Geometry: final body of the model. Coordinates: model frame, mm. A direction names the side the tool comes from. Give positions to 0.01 mm unless a question says otherwise; leave off trailing zeros. Loops run counter-clockwise (first coordinate to the right, second up) from the corner with the lowest first, then second, coordinate; pieces in that order, holes last.
1. Section B-B, the plane y = 1.15. Output: boundary loops of the cut face in (x, z).
2. Draft query along X for faces 1 (the face through (-67.25, 2, -46)), 2 (the face through (65.436, 1.61, -90.045)), 3 (the face through (-20.63, 1.57, -39.96)), 4 (the face through (20.63, 1.57, -85.24)). Return one class per face: +X half, -X half, draft (parallel to the pull), parting line (faces both ways), or undercut.
3. Section D-D, the plane x = 27.5. Output: boundary loops of the cut face in (y, z) (1 decimal), then the cut area to 3 significant figures.
4. Section A-A, the plane z = -42.6. Output: boundary loops of the cut face in (x, y) (3 decimals), then the cut area to 3 significant figures.
5. Material intervals for line 1 along X through (y, z) = (1.15, -43); line 2 along X through (y, z) = (0.65, -41); line 3 along X through (y, z) = (0.1, -69), sorted ascending.
6. Section C-C, the plane x = 44.5. Output: boundary loops of the cut face in (y, z) (3 decimals).
7. Access query for faces 5 (the face through (-1, 3.175, -29)), 6 (the face through (29.8, 1.6, -62.9)). Directions: +Z, -Z, +X, -X, +Y, -Y. A direction counts if a zero-diameter tool reaches every point of the face in a straight line with its end or side. Return the directions, or none.
8. First-contact query: P1, Ø4, axis at x = -51, z = -69.1, coming from the -Y side; P2, Ø1, axis at x = 2, y = 1, coming from the -Z side. Flat tips, straight axial feed; report the tip coordinate or a pass-through.
from build123d import *

# Parameters (mm, degrees)
SKETCH1_R           = 2.5
SKETCH1_R_2         = 12.25
BOSS_EXTRUDE1_DEPTH = 3.175
FILLET1_R           = 9.2
FILLET2_R           = 6.7


with BuildPart() as part:
    # Sketch1 → Boss-Extrude1 (new body)
    with BuildSketch(Plane(origin=(0, 0, 0), x_dir=(1, 0, 0), z_dir=(0, 1, 0))):
        with BuildLine():
            Line((-67.25, 0), (67.25, 0))
            Line((67.25, 0), (67.25, 91.408280206))
            ThreePointArc((67.25, 91.408280206), (0, 101.8), (-67.25, 91.408280206))
            Line((-67.25, 91.408280206), (-67.25, 0))
        make_face()
        with Locations(Location((-51, 69.1, 0), (0, 0, 270))):
            Circle(SKETCH1_R, mode=Mode.SUBTRACT)
        with Locations(Location((51, 69.1, 0), (0, 0, 270))):
            Circle(SKETCH1_R, mode=Mode.SUBTRACT)
        with Locations(Location((0, 12.1, 0), (0, 0, 270))):
            Circle(SKETCH1_R, mode=Mode.SUBTRACT)
        with Locations(Location((42, 42.6, 0), (0, 0, 270))):
            Circle(SKETCH1_R_2, mode=Mode.SUBTRACT)
        with BuildLine():
            Line((-14.622204703, 86.85), (14.622204703, 86.85))
            ThreePointArc((14.622204703, 86.85), (20.704967234, 85.194080433), (25.108968848, 80.683333333))
            ThreePointArc((25.108968848, 80.683333333), (29.8, 62.6), (25.108968848, 44.516666667))
            ThreePointArc((25.108968848, 44.516666667), (20.704967234, 40.005919567), (14.622204703, 38.35))
            Line((14.622204703, 38.35), (-14.622204703, 38.35))
            ThreePointArc((-14.622204703, 38.35), (-20.704967234, 40.005919567), (-25.108968848, 44.516666667))
            ThreePointArc((-25.108968848, 44.516666667), (-29.8, 62.6), (-25.108968848, 80.683333333))
            ThreePointArc((-25.108968848, 80.683333333), (-20.704967234, 85.194080433), (-14.622204703, 86.85))
        make_face(mode=Mode.SUBTRACT)
    extrude(amount=BOSS_EXTRUDE1_DEPTH)

    # Fillet1
    fillet1_edges = [part.edges().sort_by_distance(p)[0] for p in [
        (-67.25, 1.5875, -91.408280206),
        (67.25, 1.5875, -91.408280206),
    ]]
    fillet(fillet1_edges, radius=FILLET1_R)

    # Fillet2
    fillet2_edges = [part.edges().sort_by_distance(p)[0] for p in [
        (67.25, 1.5875, 0),
        (-67.25, 1.5875, 0),
    ]]
    fillet(fillet2_edges, radius=FILLET2_R)


solid = part.part
Answers below:
1. outline: (-67.25, -84.56) arc R9.2 ccw to (-60.55, -93.41) arc R222.8 ccw to (60.55, -93.41) arc R9.2 ccw to (67.25, -84.56) - (67.25, -6.7) arc R6.7 ccw to (60.55, 0) - (-60.55, 0) arc R6.7 ccw to (-67.25, -6.7) - close; hole circle Ø5 at (-51, -69.1); hole (-25.11, -80.68) arc R12 ccw to (-14.62, -86.85) - (14.62, -86.85) arc R12 ccw to (25.11, -80.68) arc R37.2 ccw to (25.11, -44.52) arc R12 ccw to (14.62, -38.35) - (-14.62, -38.35) arc R12 ccw to (-25.11, -44.52) arc R37.2 ccw to start; hole circle Ø5 at (0, -12.1); hole circle Ø24.5 at (42, -42.6); hole circle Ø5 at (51, -69.1)
2. face 1: -X half
2. face 2: +X half
2. face 3: undercut
2. face 4: undercut
3. outline: (0, -100.1) - (3.2, -100.1) - (3.2, -75.5) - (0, -75.5) - close; (0, -49.7) - (3.2, -49.7) - (3.2, 0) - (0, 0) - close
3. area: 236 mm2
4. outline: (-67.25, 0) - (-23.784, 0) - (-23.784, 3.175) - (-67.25, 3.175) - close; (23.784, 0) - (29.75, 0) - (29.75, 3.175) - (23.784, 3.175) - close; (54.25, 0) - (67.25, 0) - (67.25, 3.175) - (54.25, 3.175) - close
4. area: 198 mm2
5. line 1: x = -67.25 to -24.11, 24.11 to 29.76, 54.24 to 67.25
5. line 2: x = -67.25 to -22.14, 22.14 to 29.85, 54.15 to 67.25
5. line 3: x = -67.25 to -53.5, -48.5 to -29.25, 29.25 to 48.5, 53.5 to 67.25
6. outline: (0, -97.311) - (3.175, -97.311) - (3.175, -54.592) - (0, -54.592) - close; (0, -30.608) - (3.175, -30.608) - (3.175, 0) - (0, 0) - close
7. face 5: +Z, -Z, +X, -X, +Y
7. face 6: +Y, -Y
8. P1: passes through
8. P2: stops at z = -101.79
